Could you check a few things on this model? Use its own coordinates, in mm. Face numbers are marked on the shaded views. A direction names the side the tool comes from. Coordinates: 2 decimals unless noted, no trailing zeros. Order: outer loops, then holes, each group sorted by start corner. A loop starts at its lowest first (then second) coordinate and runs counter-clockwise, first axis right, second up. Notation, with made-up numbers: (84, 3) - (132, 3) arc R15 cw to (132, 18) - close; hole circle Ø10 at (-13, 54). An arc over 180 degrees is marked (long way). Answer as CSV lines item,"result". Start each with the question number.
1. I want a section at C-C, the plane y = 22.75. List the corners of the cut face in (x, z) for me.
2. For the marked faces 1, 2 and 3, which set-ups out of +Z, -Z, +X, -X, +Y, -Y let a thin tool reach every point of the face, with its end or its side?
3. I want a section at B-B, the plane x = 13.5. List the corners of the cut face in (y, z) for me.
4. I need wall thicknesses on probe 1 along X at (y, z) = (-0.5, 1.2); probe 2 along Y at (x, z) = (-0.5, 1.2); probe 3 along X at (y, z) = (12, 0.95). Which ranges of each line are inside material? Lowest first, please.
5. I want a section at A-A, the plane z = 0.45. List the corners of the cut face in (x, y) for me.
6. For pin 1 (1.5 mm diameter, centred on y = 9, z = 2, fed in from -X); pin 2 (1.5 mm diameter, centred on x = 2.5, z = 1.5, fed in from +Y) (3 decimals); pin 3 (1.5 mm diameter, centred on x = 2.5, z = 2, fed in from -Y), each with a flat end and sliding along its axis, tell me the tip position at first contact or that it passes through.
from build123d import *

# Parameters (mm, degrees)
CROQUIS1_W              = 3
CROQUIS1_H              = 7
CROQUIS1_W_2            = 10
CROQUIS1_H_2            = 3
SALIENTE_EXTRUIR1_DEPTH = 3


with BuildPart() as part:
    # Croquis1 → Saliente-Extruir1 (new body)
    with BuildSketch(Plane.XY):
        Polygon((20, 0), (0, 0), (0, 26), align=None)
        with Locations((-1.5, 18.5)):
            Rectangle(CROQUIS1_W, CROQUIS1_H)
        with Locations((15, -1.5)):
            Rectangle(CROQUIS1_W_2, CROQUIS1_H_2)
    extrude(amount=SALIENTE_EXTRUIR1_DEPTH)


solid = part.part
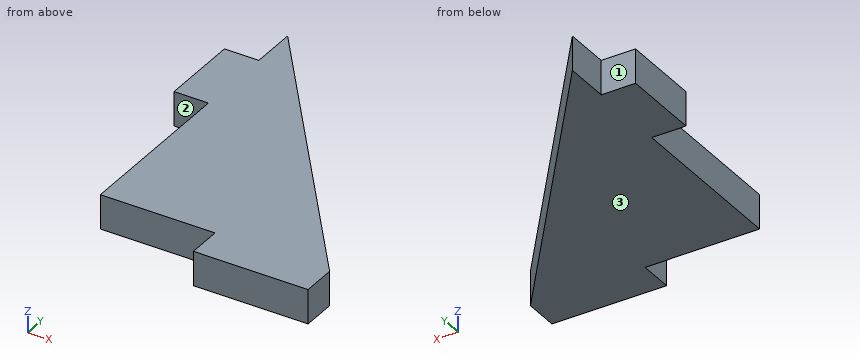
Solved:
1,outline,"(0, 0) - (2.5, 0) - (2.5, 3) - (0, 3) - close"
2,face 1,"+Z, -Z, -X, +Y"
2,face 2,"+Z, -Z, -X, -Y"
2,face 3,"-Z, +X, -X, +Y, -Y"
3,outline,"(-3, 0) - (8.45, 0) - (8.45, 3) - (-3, 3) - close"
4,probe 1,"x = 10 to 20"
4,probe 2,"y = 15 to 22"
4,probe 3,"x = 0 to 10.77"
5,outline,"(-3, 15) - (0, 15) - (0, 0) - (10, 0) - (10, -3) - (20, -3) - (20, 0) - (0, 26) - (0, 22) - (-3, 22) - close"
6,pin 1,"stops at x = 0"
6,pin 2,"stops at y = 23.725"
6,pin 3,"stops at y = 0"
